Here's how the part is built. I have some questions about the finished solid (model axes, mm). Coordinates: 2 decimals unless noted, no trailing zeros. Write each loop counter-clockwise with the first axis right and the second up, starting at its lowest first coordinate (ties: lowest second). Pieces come first, ordered by that corner, then holes.
Item 1: If we section it at C-C (y = 42.5): Please give me the cut outline in (x, z), then the cut area to 3 significant figures.
Item 2: If we section it at A-A (y = -66.5): Please give me the cut outline in (x, z), then the cut area to 3 significant figures.
Item 3: If I drill on line 1 (Y direction, x = 47, z = 1); line 2 (Y direction, x = -18.5, z = 0.8); line 3 (X direction, y = -17, z = 1.5), over which ranges is the centre line in solid material (lowest first)?
Item 4: I'm going to push flat-ended pins straight in: pin 1 Ø1 at (x, z) = (-11, 1) entering from +Y; pin 2 Ø6.5 at (x, y) = (61.22, -66.5) entering from +Z; pin 3 Ø1.5 at (y, z) = (93, 2) entering from +X; pin 4 Ø2.5 at (x, z) = (94.5, 3.5) entering from -Y. Where does each tip first touch, or does it pass through?
Item 5: If we section it at B-B (x = -35.25): Please give me the cut outline in (y, z), then the cut area to 3 significant figures.
Item 6: If we section it at D-D (x = -67): Please give me the cut outline in (y, z), then the cut area to 3 significant figures.
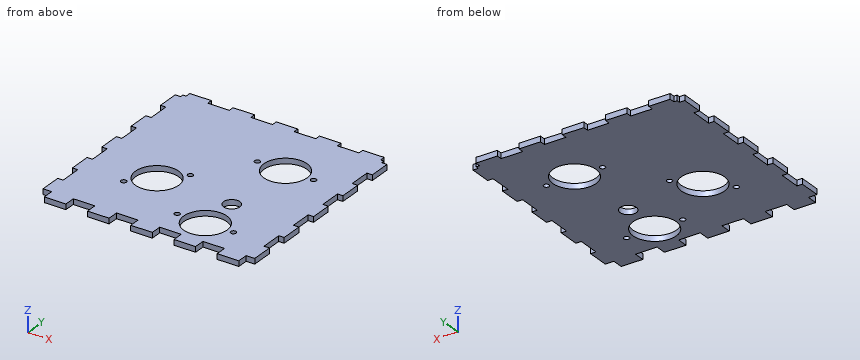
from build123d import *

# Parameters (mm, degrees)
SKETCH_1_W                       = 186
SKETCH_1_H                       = 183
SKETCH_1_R                       = 7.5
SKETCH_1_R_2                     = 20
SKETCH_1_R_3                     = 2.5
EXTRUDE_1_DEPTH                  = 5
SKETCH_2_W                       = 5
SKETCH_2_H                       = 20
EXTRUDE_2_DEPTH                  = 5
PATTERN_LINEAR_2_COUNT           = 5
PATTERN_LINEAR_2_PITCH           = 40
MIRROR_2_COPY_1_SKETCH_W         = 5
MIRROR_2_COPY_1_SKETCH_H         = 20
MIRROR_2_COPY_1_DEPTH            = 5
MIRROR_2_COPY_2_SKETCH_W         = 5
MIRROR_2_COPY_2_SKETCH_H         = 20
MIRROR_2_COPY_2_DEPTH            = 5
MIRROR_2_COPY_3_SKETCH_W         = 5
MIRROR_2_COPY_3_SKETCH_H         = 20
MIRROR_2_COPY_3_DEPTH            = 5
MIRROR_2_COPY_4_SKETCH_W         = 5
MIRROR_2_COPY_4_SKETCH_H         = 20
MIRROR_2_COPY_4_DEPTH            = 5
SKETCH_3_W                       = 20
SKETCH_3_H                       = 5
EXTRUDE_3_DEPTH                  = 5
PATTERN_LINEAR_3_COUNT           = 3
PATTERN_LINEAR_3_PITCH           = 40
PATTERN_LINEAR_4_COUNT           = 3
PATTERN_LINEAR_4_PITCH           = 40
SKETCH_4_W                       = 20
SKETCH_4_H                       = 10
EXTRUDE_4_DEPTH                  = 5
PATTERN_LINEAR_5_COUNT           = 3
PATTERN_LINEAR_5_PITCH           = 40
PATTERN_LINEAR_6_COPY_1_SKETCH_W = 20
PATTERN_LINEAR_6_COPY_1_SKETCH_H = 10
PATTERN_LINEAR_6_COPY_1_DEPTH    = 5
PATTERN_LINEAR_6_COPY_2_SKETCH_W = 20
PATTERN_LINEAR_6_COPY_2_SKETCH_H = 10
PATTERN_LINEAR_6_COPY_2_DEPTH    = 5
PATTERN_LINEAR_6_COPY_3_SKETCH_W = 20
PATTERN_LINEAR_6_COPY_3_SKETCH_H = 10
PATTERN_LINEAR_6_COPY_3_DEPTH    = 5
PATTERN_LINEAR_6_COPY_4_SKETCH_W = 20
PATTERN_LINEAR_6_COPY_4_SKETCH_H = 10
PATTERN_LINEAR_6_COPY_4_DEPTH    = 5
PATTERN_LINEAR_6_COPY_5_SKETCH_W = 20
PATTERN_LINEAR_6_COPY_5_SKETCH_H = 10
PATTERN_LINEAR_6_COPY_5_DEPTH    = 5
PATTERN_LINEAR_6_COPY_6_SKETCH_W = 20
PATTERN_LINEAR_6_COPY_6_SKETCH_H = 10
PATTERN_LINEAR_6_COPY_6_DEPTH    = 5


with BuildPart() as part:
    # 스케치1 → 보스-돌출1 (new body)
    with BuildSketch(Plane.XY):
        Rectangle(SKETCH_1_W, SKETCH_1_H)
        with Locations((35.221625496, -30.5)):
            Circle(SKETCH_1_R, mode=Mode.SUBTRACT)
        with Locations((-35.25, -28.5)):
            Circle(SKETCH_1_R_2, mode=Mode.SUBTRACT)
        with Locations((35.221625496, -66.5)):
            Circle(SKETCH_1_R_2, mode=Mode.SUBTRACT)
        with Locations((39.42261881, 36.5)):
            Circle(SKETCH_1_R_2, mode=Mode.SUBTRACT)
        with Locations((-53.634776311, -46.884776311)):
            Circle(SKETCH_1_R_3, mode=Mode.SUBTRACT)
        with Locations((-16.865223689, -10.115223689)):
            Circle(SKETCH_1_R_3, mode=Mode.SUBTRACT)
        with Locations((65.42261881, 36.5)):
            Circle(SKETCH_1_R_3, mode=Mode.SUBTRACT)
        with Locations((13.42261881, 36.5)):
            Circle(SKETCH_1_R_3, mode=Mode.SUBTRACT)
        with Locations((9.221625496, -66.5)):
            Circle(SKETCH_1_R_3, mode=Mode.SUBTRACT)
        with Locations((61.221625496, -66.5)):
            Circle(SKETCH_1_R_3, mode=Mode.SUBTRACT)
    extrude(amount=EXTRUDE_1_DEPTH)

    # 스케치2 → 보스-돌출2 (add)
    with BuildSketch(Plane.XY.offset(5)):
        with Locations((95.5, -81.5)):
            Rectangle(SKETCH_2_W, SKETCH_2_H)
    extrude_2 = extrude(amount=-EXTRUDE_2_DEPTH)

    # 선형 패턴2: 보스-돌출2 ×5
    with Locations(*[(0, i * PATTERN_LINEAR_2_PITCH, 0) for i in range(1, PATTERN_LINEAR_2_COUNT)]):
        add(extrude_2)

    # 대칭 복사2: 보스-돌출2 across plane
    add(extrude_2.mirror(Plane(origin=(0, 0, 0), x_dir=(0, 0, 1), z_dir=(1, 0, 0))))

    # 대칭 복사2 copy 1 sketch → 대칭 복사2 copy 1 (add)
    with BuildSketch(Plane(origin=(0, 40, 5), x_dir=(-1, 0, 0), z_dir=(0, 0, 1))):
        with Locations((95.5, 81.5)):
            Rectangle(MIRROR_2_COPY_1_SKETCH_W, MIRROR_2_COPY_1_SKETCH_H)
    extrude(amount=-MIRROR_2_COPY_1_DEPTH)

    # 대칭 복사2 copy 2 sketch → 대칭 복사2 copy 2 (add)
    with BuildSketch(Plane(origin=(0, 80, 5), x_dir=(-1, 0, 0), z_dir=(0, 0, 1))):
        with Locations((95.5, 81.5)):
            Rectangle(MIRROR_2_COPY_2_SKETCH_W, MIRROR_2_COPY_2_SKETCH_H)
    extrude(amount=-MIRROR_2_COPY_2_DEPTH)

    # 대칭 복사2 copy 3 sketch → 대칭 복사2 copy 3 (add)
    with BuildSketch(Plane(origin=(0, 120, 5), x_dir=(-1, 0, 0), z_dir=(0, 0, 1))):
        with Locations((95.5, 81.5)):
            Rectangle(MIRROR_2_COPY_3_SKETCH_W, MIRROR_2_COPY_3_SKETCH_H)
    extrude(amount=-MIRROR_2_COPY_3_DEPTH)

    # 대칭 복사2 copy 4 sketch → 대칭 복사2 copy 4 (add)
    with BuildSketch(Plane(origin=(0, 160, 5), x_dir=(-1, 0, 0), z_dir=(0, 0, 1))):
        with Locations((95.5, 81.5)):
            Rectangle(MIRROR_2_COPY_4_SKETCH_W, MIRROR_2_COPY_4_SKETCH_H)
    extrude(amount=-MIRROR_2_COPY_4_DEPTH)

    # 스케치3 → 보스-돌출3 (add)
    with BuildSketch(Plane.XY.offset(5)):
        with Locations((0, 94)):
            Rectangle(SKETCH_3_W, SKETCH_3_H)
    extrude_3 = extrude(amount=-EXTRUDE_3_DEPTH)

    # 선형 패턴3: 보스-돌출3 ×3
    with Locations(*[(i * PATTERN_LINEAR_3_PITCH, 0, 0) for i in range(1, PATTERN_LINEAR_3_COUNT)]):
        add(extrude_3)

    # 선형 패턴4: 보스-돌출3 ×3
    with Locations(*[(-i * PATTERN_LINEAR_4_PITCH, 0, 0) for i in range(1, PATTERN_LINEAR_4_COUNT)]):
        add(extrude_3)

    # 스케치4 → 보스-돌출4 (add)
    with BuildSketch(Plane.XY.offset(5)):
        with Locations((0, -96.5)):
            Rectangle(SKETCH_4_W, SKETCH_4_H)
    extrude_4 = extrude(amount=-EXTRUDE_4_DEPTH)

    # 선형 패턴5: 보스-돌출4 ×3
    with Locations(*[(i * PATTERN_LINEAR_5_PITCH, 0, 0) for i in range(1, PATTERN_LINEAR_5_COUNT)]):
        add(extrude_4)

    # 선형 패턴6 copy 1 sketch → 선형 패턴6 copy 1 (add)
    with BuildSketch(Plane.XY.offset(5)):
        with Locations((0, -96.5)):
            Rectangle(PATTERN_LINEAR_6_COPY_1_SKETCH_W, PATTERN_LINEAR_6_COPY_1_SKETCH_H)
    extrude(amount=-PATTERN_LINEAR_6_COPY_1_DEPTH)

    # 선형 패턴6 copy 2 sketch → 선형 패턴6 copy 2 (add)
    with BuildSketch(Plane(origin=(-40, 0, 5), x_dir=(1, 0, 0), z_dir=(0, 0, 1))):
        with Locations((0, -96.5)):
            Rectangle(PATTERN_LINEAR_6_COPY_2_SKETCH_W, PATTERN_LINEAR_6_COPY_2_SKETCH_H)
    extrude(amount=-PATTERN_LINEAR_6_COPY_2_DEPTH)

    # 선형 패턴6 copy 3 sketch → 선형 패턴6 copy 3 (add)
    with BuildSketch(Plane(origin=(40, 0, 5), x_dir=(1, 0, 0), z_dir=(0, 0, 1))):
        with Locations((0, -96.5)):
            Rectangle(PATTERN_LINEAR_6_COPY_3_SKETCH_W, PATTERN_LINEAR_6_COPY_3_SKETCH_H)
    extrude(amount=-PATTERN_LINEAR_6_COPY_3_DEPTH)

    # 선형 패턴6 copy 4 sketch → 선형 패턴6 copy 4 (add)
    with BuildSketch(Plane.XY.offset(5)):
        with Locations((0, -96.5)):
            Rectangle(PATTERN_LINEAR_6_COPY_4_SKETCH_W, PATTERN_LINEAR_6_COPY_4_SKETCH_H)
    extrude(amount=-PATTERN_LINEAR_6_COPY_4_DEPTH)

    # 선형 패턴6 copy 5 sketch → 선형 패턴6 copy 5 (add)
    with BuildSketch(Plane(origin=(-40, 0, 5), x_dir=(1, 0, 0), z_dir=(0, 0, 1))):
        with Locations((0, -96.5)):
            Rectangle(PATTERN_LINEAR_6_COPY_5_SKETCH_W, PATTERN_LINEAR_6_COPY_5_SKETCH_H)
    extrude(amount=-PATTERN_LINEAR_6_COPY_5_DEPTH)

    # 선형 패턴6 copy 6 sketch → 선형 패턴6 copy 6 (add)
    with BuildSketch(Plane(origin=(-80, 0, 5), x_dir=(1, 0, 0), z_dir=(0, 0, 1))):
        with Locations((0, -96.5)):
            Rectangle(PATTERN_LINEAR_6_COPY_6_SKETCH_W, PATTERN_LINEAR_6_COPY_6_SKETCH_H)
    extrude(amount=-PATTERN_LINEAR_6_COPY_6_DEPTH)


solid = part.part
Answer list:
1. outline: (-98, 0) - (20.34, 0) - (20.34, 5) - (-98, 5) - close; (58.5, 0) - (98, 0) - (98, 5) - (58.5, 5) - close
1. area: 789 mm2
2. outline: (-93, 0) - (6.72, 0) - (6.72, 5) - (-93, 5) - close; (11.72, 0) - (15.22, 0) - (15.22, 5) - (11.72, 5) - close; (55.22, 0) - (58.72, 0) - (58.72, 5) - (55.22, 5) - close; (63.72, 0) - (93, 0) - (93, 5) - (63.72, 5) - close
2. area: 680 mm2
3. line 1: y = -101.5 to -82.66, -50.34 to 17.99, 55.01 to 96.5
3. line 2: y = -91.5 to -39.43, -17.57 to -12.01, -8.22 to 91.5
3. line 3: x = -93 to -51.61, -18.89 to 93
4. pin 1: stops at y = 91.5
4. pin 2: stops at z = 5
4. pin 3: stops at x = 90
4. pin 4: stops at y = -91.5
5. outline: (-101.5, 0) - (-48.5, 0) - (-48.5, 5) - (-101.5, 5) - close; (-8.5, 0) - (96.5, 0) - (96.5, 5) - (-8.5, 5) - close
5. area: 790 mm2
6. outline: (-91.5, 0) - (91.5, 0) - (91.5, 5) - (-91.5, 5) - close
6. area: 915 mm2
